The model under review builds one solid part; all positions refer to its coordinate system, in mm. A direction names the side the tool comes from. Round coordinates to 2 decimals unless told otherwise and drop trailing zeros. Order: outer loops, then holes, each group sorted by start corner. A loop starts at its lowest first (then second) coordinate and runs counter-clockwise, first axis right, second up. Notation, with made-up numbers: (-0.5, 70.25) -> (49.5, 70.25) arc R10 ccw to (49.5, 81.25) -> close; hole circle Ø8 at (-39, 74). An arc over 180 degrees is marked (long way). Use a Markdown table: item, result. Add a question column.
```python
from build123d import *

# Parameters (mm, degrees)
F1_DEPTH       = 17.78
F0_W           = 3.175
F0_H           = 0.3175
F2_DEPTH       = 17.78
F5_D           = 6.6
F5_DEPTH       = 12.7
F5_TIP         = 1.9828400428
F5_ON_F3_D     = 6.6
F5_ON_F3_DEPTH = 12.7
F5_ON_F3_TIP   = 1.9828400428
F6_W           = 12.7
F6_H           = 3.175
F8_DEPTH       = 12.7
F7_W           = 12.7
F7_H           = 3.175
F9_DEPTH       = 12.7


with BuildPart() as f1:
    # F0 (on Right) → F1 (new body)
    with BuildSketch(Plane.YZ):
        Polygon((-11.4516578615, 40.005), (-17.8016578615, 40.005), (-17.8016578615, 27.305), (-30.5016578615, 27.305), (-30.5016578615, -40.005), (-17.5, -40.005), (-17.5, -33.505), (-17.5, -32.505), (17.5, -32.505), (17.5, -33.505), (14, -40.005), (29.4423421385, -40.005), (29.4423421385, 27.305), (16.7423421385, 27.305), (16.7423421385, 40.005), (10.3923421385, 40.005), (1.0578421385, 40.005), (-0.5296578615, 40.005), (-2.1171578615, 40.005), align=None)
    extrude(amount=F1_DEPTH)

    # F0 (on Right) → F2 (join, through all)
    with BuildSketch(Plane.YZ):
        with BuildLine():
            ThreePointArc((10.3923421385, 40.005), (5.8318480853, 41.5948737402), (1.0578421385, 42.3260862531))
            Line((1.0578421385, 42.3260862531), (1.0578421385, 40.005))
            Line((1.0578421385, 40.005), (10.3923421385, 40.005))
        make_face()
        with BuildLine():
            Line((-2.1171578615, 42.3260862531), (-2.1171578615, 40.005))
            Line((-2.1171578615, 40.005), (-0.5296578615, 40.005))
            Line((-0.5296578615, 40.005), (1.0578421385, 40.005))
            Line((1.0578421385, 40.005), (1.0578421385, 42.3260862531))
            ThreePointArc((1.0578421385, 42.3260862531), (-0.5296578615, 42.3739277182), (-2.1171578615, 42.3260862531))
        make_face()
        with BuildLine():
            ThreePointArc((-2.1171578615, 42.3260862531), (-6.8911638083, 41.5948737402), (-11.4516578615, 40.005))
            Line((-11.4516578615, 40.005), (-2.1171578615, 40.005))
            Line((-2.1171578615, 40.005), (-2.1171578615, 42.3260862531))
        make_face()
        with BuildLine():
            Line((-2.1171578615, 44.7675), (-2.1171578615, 42.3260862531))
            ThreePointArc((-2.1171578615, 42.3260862531), (-0.5296578615, 42.3739277182), (1.0578421385, 42.3260862531))
            Line((1.0578421385, 42.3260862531), (1.0578421385, 44.7675))
            Line((1.0578421385, 44.7675), (-2.1171578615, 44.7675))
        make_face()
        with Locations((-0.5296578615, 44.92625)):
            Rectangle(F0_W, F0_H)
        Polygon((-2.7487089392, 44.7675), (-2.1171578615, 44.7675), (-2.1171578615, 45.085), (1.0578421385, 45.085), (1.0578421385, 44.7675), (1.628424623, 44.7675), (1.628424623, 46.0375), (-2.7487089392, 46.0375), align=None)
    extrude(amount=F2_DEPTH)

    # F5
    with Locations(Plane.XY.offset(27.305)):
        with Locations((8.89, 23.0923421385)):
            Hole(F5_D / 2, depth=F5_DEPTH)
            with Locations((0, 0, -(F5_DEPTH + F5_TIP / 2))):  # 118° drill point
                Cone(0, F5_D / 2, F5_TIP, mode=Mode.SUBTRACT)

    # F5 on F3
    with Locations(Plane.XY.offset(27.305)):
        with Locations((8.89, -24.1516578615)):
            Hole(F5_ON_F3_D / 2, depth=F5_ON_F3_DEPTH)
            with Locations((0, 0, -(F5_ON_F3_DEPTH + F5_ON_F3_TIP / 2))):  # 118° drill point
                Cone(0, F5_ON_F3_D / 2, F5_ON_F3_TIP, mode=Mode.SUBTRACT)

    # F6 (on face) → F8 (cut)
    with BuildSketch(Plane.XZ.offset(30.5016578615)):
        with Locations((8.89, 16.1925)):
            Rectangle(F6_W, F6_H)
    extrude(amount=-F8_DEPTH, mode=Mode.SUBTRACT)

    # F7 (on face) → F9 (cut)
    with BuildSketch(Plane(origin=(0, 29.4423421385, 0), x_dir=(-1, 0, 0), z_dir=(0, 1, 0))):
        with Locations((-8.89, 16.1925)):
            Rectangle(F7_W, F7_H)
    extrude(amount=-F9_DEPTH, mode=Mode.SUBTRACT)


solid = f1.part
```
Q1. Insertion check: pin 1 (0.6 mm diameter, centred on x = 9, z = 45.5, fed in from -Y); pin 2 (0.5 mm diameter, centred on x = 7.5, y = -2.5, fed in from -Z) (3 decimals); pin 3 (4 mm diameter, centred on x = 11.5, y = -21.5, fed in from +Z) (3 decimals). Each pin has a flat end and moves straight along its axis. Give the tip position at first contact, or say it passes through.
Q2. Machinability: for faces 1 (the flat face through (9, 1.058, 44)), 2 (the flat face through (6, -21, 17.78)), 3 (the flat face through (9, 14, 40.005)), 4 (the flat face through (15.24, 23, 16)), 5 (the flat face through (9, -15, 40.005)), which of the approach directions +Z, -Z, +X, -X, +Y, -Y give a long, thin tool a straight path to every point of the face, cutting with its end or side? Answer none if there is none.
Q3. Mouldability with a two-part tool opening along Z and no side actions: class faces 6 (the flat face through (6, 20, 17.78)), 7 (the flat face through (15.24, -24, 16)), 8 (the conical face through (8.766, -24.711, 12.967)), 9 (the cylindrical face through (9.32, -20.88, 22.48)) as pulls with the +Z half, pulls with the -Z half, needs draft (parallel to the pull), parting line crosses it, or undercut.
Q4. Add section A-A (x = 16.75). Write out the cut boundary in (y, z) (1 decimal).
Q5. Add section B-B (z = 25). Write out the cut boundary in (x, y), then the cut area to 3 significant figures.
Q6. Wall thickness on line 1 (Y direction, x = 8.89, z = 21); line 2 (Y direction, x = 11.5, z = -33.5); line 3 (Y direction, x = 6.5, z = 20): over which ranges is each line inside the solid? List them lowest first. Write a range as [from, to].
Q7. Add section C-C (x = 10). State how many separate pieces and enclosed holes the cut face has, then the cut area to 3 significant figures.
Report:
| question | item | result |
|---|---|---|
| 1 | pin 1 | stops at y = -2.75 |
| 1 | pin 2 | stops at z = -32.505 |
| 1 | pin 3 | stops at z = 27.305 |
| 2 | face 1 | +X, -X, +Y |
| 2 | face 2 | -Y |
| 2 | face 3 | +Z, +X, -X, +Y |
| 2 | face 4 | +Y |
| 2 | face 5 | +Z, +X, -X, -Y |
| 3 | face 6 | undercut |
| 3 | face 7 | undercut |
| 3 | face 8 | pulls with the +Z half |
| 3 | face 9 | needs draft |
| 4 | outline | (-30.5, -40) -> (-17.5, -40) -> (-17.5, -32.5) -> (17.5, -32.5) -> (17.5, -33.5) -> (14, -40) -> (29.4, -40) -> (29.4, 27.3) -> (16.7, 27.3) -> (16.7, 40) -> (10.4, 40) arc R26.4 ccw to (1.1, 42.3) -> (1.1, 44.8) -> (1.6, 44.8) -> (1.6, 46) -> (-2.7, 46) -> (-2.7, 44.8) -> (-2.1, 44.8) -> (-2.1, 42.3) arc R26.4 ccw to (-11.5, 40) -> (-17.8, 40) -> (-17.8, 27.3) -> (-30.5, 27.3) -> close |
| 5 | outline | (0, -30.5) -> (17.78, -30.5) -> (17.78, 29.44) -> (0, 29.44) -> close; hole circle Ø6.6 at (8.89, -24.15); hole circle Ø6.6 at (8.89, 23.09) |
| 5 | area | 997 mm² |
| 6 | line 1 | y = [-30.5, -27.45], [-20.85, 19.79], [26.39, 29.44] |
| 6 | line 2 | y = [-30.5, -17.5], [17.5, 29.44] |
| 6 | line 3 | y = [-30.5, -26.43], [-21.88, 20.82], [25.37, 29.44] |
| 7 | separate pieces | 3 |
| 7 | enclosed holes | 0 |
| 7 | area | 4,060 mm² |
